The drawing under review shows one solid part. Ordinate dimensions are in mm from its lowest x, y, z. Coordinates: 2 decimals unless noted, no trailing zeros. Write each loop counter-clockwise with the first axis right and the second up, starting at its lowest first coordinate (ties: lowest second). Pieces come first, ordered by that corner, then holes.
1) For P1, Ø1, axis at x = 5.5, z = 11, coming from the -Y side; P2, Ø1.5, axis at x = 1, z = 15.5, coming from the -Y side, all flat-tipped, find the tip position at first contact; note any pin that passes through.
2) Add section A-A, the plane z = 16.5. State the section outline as (x, y) points, then the cut area to 3 significant figures.
3) For line 1 (Z direction, x = 5.3, y = 4.7); line 2 (Z direction, x = 2.7, y = 5.7); line 3 (Y direction, x = 2.85, z = 9), list the stretches that pass through material, from the lowest coordinate up.
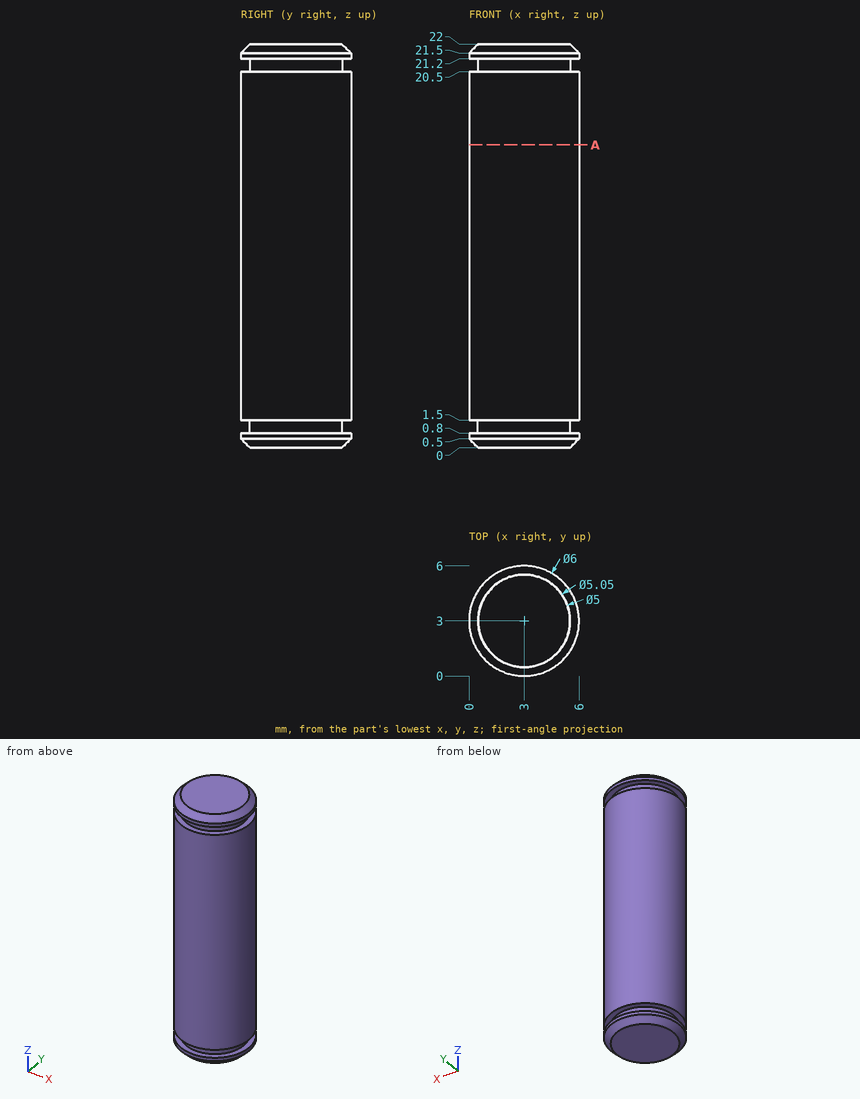
Geometry results:
1. P1: stops at y = 0.76
1. P2: stops at y = 0.27
2. outline: circle Ø6 at (3, 3)
2. area: 28.3 mm2
3. line 1: z = 0.36 to 0.8, 1.5 to 20.5, 21.2 to 21.64
3. line 2: z = 0.22 to 0.8, 1.5 to 20.5, 21.2 to 21.78
3. line 3: y = 0 to 6
